Read the model definition and answer for the solid it produces. Units are mm, in the model's axes. A direction names the side the tool comes from. Coordinates: 2 decimals unless noted, no trailing zeros. Order: outer loops, then holes, each group sorted by start corner. A loop starts at its lowest first (then second) coordinate and runs counter-clockwise, first axis right, second up. Notation, with made-up numbers: (-27.75, -2.75) -> (9.25, -2.75) arc R28 ccw to (9.25, 28.25) -> close; hole circle Ø1 at (-29, 10). An arc over 180 degrees is marked (long way). Use CSV: the item, a comma, the result in double quotes.
```python
from build123d import *

# Parameters (mm, degrees)
SKETCH_1_W          = 60
SKETCH_1_H          = 50
SKETCH_1_R          = 1.6
SKETCH_1_W_2        = 44
SKETCH_1_H_2        = 34
EXTRUDE_1_DEPTH     = 8
SKETCH_2_R          = 1.6
CUT_EXTRUDE_1_DEPTH = 10
CUT_EXTRUDE_START   = -40
SKETCH_2_2_R        = 1.6
CUT_EXTRUDE_2_DEPTH = 10


with BuildPart() as part:
    # 草图1 → 凸台-拉伸1 (new body)
    with BuildSketch(Plane(origin=(0, 0, 0), x_dir=(0, 0, -1), z_dir=(1, 0, 0))):
        with Locations((30, 25)):
            Rectangle(SKETCH_1_W, SKETCH_1_H)
        with Locations((15, 46)):
            Circle(SKETCH_1_R, mode=Mode.SUBTRACT)
        with Locations((45, 46)):
            Circle(SKETCH_1_R, mode=Mode.SUBTRACT)
        with Locations((15, 4)):
            Circle(SKETCH_1_R, mode=Mode.SUBTRACT)
        with Locations((45, 4)):
            Circle(SKETCH_1_R, mode=Mode.SUBTRACT)
        with Locations((30, 25)):
            Rectangle(SKETCH_1_W_2, SKETCH_1_H_2, mode=Mode.SUBTRACT)
    extrude(amount=EXTRUDE_1_DEPTH)

    # 草图2 → 切除-拉伸1 (cut)
    with BuildSketch(Plane.XZ):
        with Locations(Location((4, -5, 0), (0, 0, 270))):
            Circle(SKETCH_2_R)
        with Locations(Location((4, -30, 0), (0, 0, 270))):
            Circle(SKETCH_2_R)
        with Locations(Location((4, -55, 0), (0, 0, 270))):
            Circle(SKETCH_2_R)
    extrude(amount=-CUT_EXTRUDE_1_DEPTH, mode=Mode.SUBTRACT)

    # 草图2<2> → 切除-拉伸2 (cut)
    with BuildSketch(Plane.XZ.offset(CUT_EXTRUDE_START)):
        with Locations(Location((4, -5, 0), (0, 0, 270))):
            Circle(SKETCH_2_2_R)
        with Locations(Location((4, -30, 0), (0, 0, 270))):
            Circle(SKETCH_2_2_R)
        with Locations(Location((4, -55, 0), (0, 0, 270))):
            Circle(SKETCH_2_2_R)
    extrude(amount=-CUT_EXTRUDE_2_DEPTH, mode=Mode.SUBTRACT)


solid = part.part
```
Item 1: Each of these flat-tipped pins is pushed along its axis until it touches: P1, Ø3.5, axis at x = 4, z = -54.5, coming from the -Y side; P2, Ø1.9, axis at x = 4, z = -55, coming from the +Y side; P3, Ø3, axis at x = 4, z = -5, coming from the -Y side. Where does it stop, or does it pass through?
Return value:
P1,"stops at y = 0"
P2,"stops at y = 40"
P3,"stops at y = 10"
Item 2: Find section A-A, the plane y = 46. Give the vertices of the cut face in (x, z), then the cut area to 3 significant figures.
Return value:
outline,"(0, -60) -> (8, -60) -> (8, -46.6) -> (0, -46.6) -> close; (0, -43.4) -> (8, -43.4) -> (8, -16.6) -> (0, -16.6) -> close; (0, -13.4) -> (8, -13.4) -> (8, 0) -> (0, 0) -> close; hole circle Ø3.2 at (4, -55); hole circle Ø3.2 at (4, -30); hole circle Ø3.2 at (4, -5)"
area,"405 mm^2"
Item 3: Find section B-B, the plane z = -38.5. Give the vertices of the cut face in (x, y), then the cut area to 3 significant figures.
Return value:
outline,"(0, 0) -> (8, 0) -> (8, 8) -> (0, 8) -> close; (0, 42) -> (8, 42) -> (8, 50) -> (0, 50) -> close"
area,"128 mm^2"
Item 4: Find section C-C, the plane y = 15. Give the vertices of the cut face in (x, z), then the cut area to 3 significant figures.
Return value:
outline,"(0, -60) -> (8, -60) -> (8, -52) -> (0, -52) -> close; (0, -8) -> (8, -8) -> (8, 0) -> (0, 0) -> close"
area,"128 mm^2"
Item 5: Find section D-D, the plane z = -15. Give the vertices of the cut face in (x, y), then the cut area to 3 significant figures.
Return value:
outline,"(0, 0) -> (8, 0) -> (8, 2.4) -> (0, 2.4) -> close; (0, 5.6) -> (8, 5.6) -> (8, 8) -> (0, 8) -> close; (0, 42) -> (8, 42) -> (8, 44.4) -> (0, 44.4) -> close; (0, 47.6) -> (8, 47.6) -> (8, 50) -> (0, 50) -> close"
area,"76.8 mm^2"
Item 6: A tool of negligible diameter and unlimited length cuts with its end or side. For faces 1 (the flat face through (2, 0, -30)), 2 (the cylindrical face through (3.39, 4.93, -6.48)), 3 (the flat face through (4, 40, -55)), 4 (the flat face through (2, 42, -30)), from which of +Z, -Z, +X, -X, +Y, -Y can it reach the whole face along a straight path? Write none if from no direction.
Return value:
face 1,"+Z, -Z, +X, -X, -Y"
face 2,"-Y"
face 3,"+Y"
face 4,"+X, -X"
Item 7: Straight lines are drawn through the part: line 1 along Y through (x, z) = (2.5, -15); line 2 along Y through (x, z) = (4.5, -26); line 3 along X through (y, z) = (5.75, -30). For each, find the intervals that lie inside material, in ascending order.
Return value:
line 1,"y = 0 to 2.4, 5.6 to 8, 42 to 44.4, 47.6 to 50"
line 2,"y = 0 to 8, 42 to 50"
line 3,"x = 0 to 2.4, 5.6 to 8"
Item 8: The mould has two halves that part along Z. Classify faces 5 (the flat face through (4, 25, 0)), 6 (the flat face through (4, 25, -52)), 7 (the flat face through (8, 48, -30)), 8 (the cylindrical face through (3.94, 4.07, -13.4)): +Z half, -Z half, draft (parallel to the pull), parting line (faces both ways), or undercut.
Return value:
face 5,"+Z half"
face 6,"undercut"
face 7,"draft"
face 8,"undercut"
